Geometry: final body of the model. Coordinates: model frame, mm. Face numbers are marked on the shaded views. A direction names the side the tool comes from. Round coordinates to 2 decimals unless told otherwise and drop trailing zeros. Write each loop counter-clockwise with the first axis right and the second up, starting at its lowest first coordinate (ties: lowest second). Pieces come first, ordered by that corner, then holes. Notation, with made-up numbers: (76.25, 75) - (82.25, 75) arc R30 cw to (82.25, 112) - close; hole circle Ø7 at (33, 25.25). An arc over 180 degrees is marked (long way). Write each question's results on one line, items separated by ' | '.
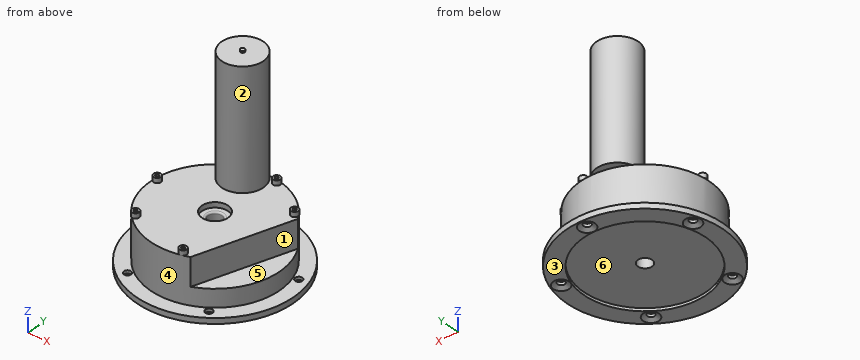
from build123d import *

# Parameters (mm, degrees)
FILLET1_R          = 1.524
SKETCH3_R          = 56.007
EXTRUDE1_DEPTH     = 2.6416
EXTRUDE3_REACH     = 7.08
SKETCH5_R          = 3.2639
CHAMFER1_SIZE      = 3.9878
CHAMFER1_SIZE2     = 2.302357403
EXTRUDE4_DEPTH     = 25.4
SKETCH7_R          = 19.05
EXTRUDE5_DEPTH     = 107.95
SKETCH9_R          = 3.3655
EXTRUDE6_DEPTH     = 4.445
SKETCH10_R         = 1.9685
EXTRUDE7_DEPTH     = 24.765
CUT_EXTRUDE1_START = 1.5875
SKETCH15_R         = 1.9685
CUT_EXTRUDE1_DEPTH = 24.1775


with BuildPart() as part:
    # Sketch2 → Revolve1 (revolve)
    with BuildSketch(Plane(origin=(0, 0, 0), x_dir=(0, 0, -1), z_dir=(1, 0, 0))):
        Polygon((0, 6.477), (0, 71.8185), (-5.08, 71.8185), (-5.08, 58.9915), (-46.609, 58.9915), (-46.609, 11.938), (-41.8465, 11.938), (-41.8465, 6.477), align=None)
    revolve(axis=Axis((0, 0, 46.609), (0, 0, -1)))

    # Fillet1
    fillet1_edges = [part.edges().sort_by_distance(p)[0] for p in [
        (0, -6.477, 41.8465),
    ]]
    fillet(fillet1_edges, radius=FILLET1_R)

    # Sketch3 → Extrude1 (cut)
    with BuildSketch(Plane(origin=(0, 0, 0), x_dir=(-1, 0, 0), z_dir=(0, 0, -1))):
        Circle(SKETCH3_R)
    extrude(amount=-EXTRUDE1_DEPTH, mode=Mode.SUBTRACT)

    # Sketch5 → Extrude3 (cut, up to next)
    with BuildSketch(Plane.XY.offset(5.08), mode=Mode.PRIVATE) as extrude3_sk1:
        with Locations((0, 63.5)):
            Circle(SKETCH5_R)
    extrude3_tool1 = extrude(extrude3_sk1.sketch, amount=-EXTRUDE3_REACH, mode=Mode.PRIVATE) & part.part
    add(extrude3_tool1.solids().sort_by_distance((0, 63.5, 5.08))[0], mode=Mode.SUBTRACT)
    # Sketch5 → Extrude3 (cut, up to next)
    with BuildSketch(Plane.XY.offset(5.08), mode=Mode.PRIVATE) as extrude3_sk2:
        with Locations((60.392088785, 19.622579143)):
            Circle(SKETCH5_R)
    extrude3_tool2 = extrude(extrude3_sk2.sketch, amount=-EXTRUDE3_REACH, mode=Mode.PRIVATE) & part.part
    add(extrude3_tool2.solids().sort_by_distance((60.392089, 19.622579, 5.08))[0], mode=Mode.SUBTRACT)
    # Sketch5 → Extrude3 (cut, up to next)
    with BuildSketch(Plane.XY.offset(5.08), mode=Mode.PRIVATE) as extrude3_sk3:
        with Locations((37.324363521, -51.372579143)):
            Circle(SKETCH5_R)
    extrude3_tool3 = extrude(extrude3_sk3.sketch, amount=-EXTRUDE3_REACH, mode=Mode.PRIVATE) & part.part
    add(extrude3_tool3.solids().sort_by_distance((37.324364, -51.372579, 5.08))[0], mode=Mode.SUBTRACT)
    # Sketch5 → Extrude3 (cut, up to next)
    with BuildSketch(Plane.XY.offset(5.08), mode=Mode.PRIVATE) as extrude3_sk4:
        with Locations((-37.324363521, -51.372579143)):
            Circle(SKETCH5_R)
    extrude3_tool4 = extrude(extrude3_sk4.sketch, amount=-EXTRUDE3_REACH, mode=Mode.PRIVATE) & part.part
    add(extrude3_tool4.solids().sort_by_distance((-37.324364, -51.372579, 5.08))[0], mode=Mode.SUBTRACT)
    # Sketch5 → Extrude3 (cut, up to next)
    with BuildSketch(Plane.XY.offset(5.08), mode=Mode.PRIVATE) as extrude3_sk5:
        with Locations((-60.392088785, 19.622579143)):
            Circle(SKETCH5_R)
    extrude3_tool5 = extrude(extrude3_sk5.sketch, amount=-EXTRUDE3_REACH, mode=Mode.PRIVATE) & part.part
    add(extrude3_tool5.solids().sort_by_distance((-60.392089, 19.622579, 5.08))[0], mode=Mode.SUBTRACT)

    # Chamfer1
    chamfer1_edges = [part.edges().sort_by_distance(p)[0] for p in [
        (-3.2639, 63.5, 0),
        (57.128188785, 19.622579143, 0),
        (34.060463521, -51.372579143, 0),
        (-40.588263521, -51.372579143, 0),
        (-63.655988785, 19.622579143, 0),
    ]]
    chamfer1_side = [part.faces().sort_by_distance(p)[0] for p in [
        (0, -69.787166065, 0),
    ]]
    chamfer(chamfer1_edges, length=CHAMFER1_SIZE, length2=CHAMFER1_SIZE2, reference=chamfer1_side[0])

    # Sketch6 → Extrude4 (cut)
    with BuildSketch(Plane.XY.offset(46.609)):
        Polygon((50.54556585, 30.416160921), (23.014050942, -54.317129264), (47.170886456, -62.166160921), (74.702401364, 22.567129264), align=None)
    extrude(amount=-EXTRUDE4_DEPTH, mode=Mode.SUBTRACT)

    # Sketch7 → Extrude5 (add)
    with BuildSketch(Plane.XY.offset(46.609)):
        with Locations((-12.023794238, 44.70269952)):
            Circle(SKETCH7_R)
    extrude(amount=EXTRUDE5_DEPTH)

    # Sketch9 → Extrude6 (add)
    with BuildSketch(Plane.XY.offset(46.609)):
        with Locations((45.289737364, 33.164222372)):
            Circle(SKETCH9_R)
        Polygon((46.260636305, 31.696529201), (47.046246406, 33.271198934), (46.075347464, 34.738892106), (44.318838422, 34.631915543), (43.533228322, 33.057245809), (44.504127263, 31.589552638), align=None, mode=Mode.SUBTRACT)
        with Locations((10.504871796, 55.142303403)):
            Circle(SKETCH9_R)
        Polygon((12.215906667, 54.731052055), (11.716543346, 56.418477394), (10.005508475, 56.829728741), (8.793836925, 55.55355475), (9.293200246, 53.866129412), (11.004235117, 53.454878064), align=None, mode=Mode.SUBTRACT)
        with Locations((15.674172573, -53.901264087)):
            Circle(SKETCH9_R)
        Polygon((13.962925135, -54.311630029), (15.173936185, -55.588430811), (16.885183622, -55.178064869), (17.38542001, -53.490898144), (16.174408961, -52.214097362), (14.463161523, -52.624463305), align=None, mode=Mode.SUBTRACT)
        with Locations((-56.011502863, 3.706413765)):
            Circle(SKETCH9_R)
        Polygon((-55.811839617, 5.454813773), (-57.425830063, 4.753527212), (-57.625493309, 3.005127204), (-56.211166109, 1.958013757), (-54.597175663, 2.659300318), (-54.397512417, 4.407700326), align=None, mode=Mode.SUBTRACT)
        with Locations((-39.544118158, -39.840791598)):
            Circle(SKETCH9_R)
        Polygon((-40.732661518, -38.543050222), (-41.262266837, -40.221229654), (-40.073723476, -41.51897103), (-38.355574797, -41.138532974), (-37.825969478, -39.460353542), (-39.014512839, -38.162612166), align=None, mode=Mode.SUBTRACT)
    extrude(amount=EXTRUDE6_DEPTH)

    # Sketch10 → Extrude7 (add)
    with BuildSketch(Plane.XY.offset(154.559)):
        with Locations((-12.023794238, 44.70269952)):
            Circle(SKETCH10_R)
    extrude(amount=EXTRUDE7_DEPTH)

    # Sketch15 → Cut-Extrude1 (cut, through all)
    with BuildSketch(Plane.XY.offset(154.559).offset(CUT_EXTRUDE1_START)):
        with Locations((-12.023794238, 44.70269952)):
            Circle(SKETCH15_R)
    extrude(amount=CUT_EXTRUDE1_DEPTH, mode=Mode.SUBTRACT)


solid = part.part
Q1. Mould query, pull axis X, two halves, no side actions, for the marked faces 4, 5 and 6. Classes: pulls with the +X half, pulls with the -X half, needs draft (parallel to the pull), parting line crosses it, or undercut.
Answer block:
face 4: parting line crosses it | face 5: needs draft | face 6: undercut
Q2. Section query C-C, the plane z = 88.5. Return loops of the section in (x, y).
Answer block:
outline: circle Ø38.1 at (-12.02, 44.7)
Q3. Access query for the marked faces 1, 2 and 3. Directions: +Z, -Z, +X, -X, +Y, -Y. A direction counts if a zero-diameter tool reaches every point of the face in a straight line with its end or side. Return the directions, or none.
Answer block:
face 1: +Z, +X, -Y | face 2: +Z | face 3: -Z, +X, -X, +Y, -Y
Q4. Section query B-B, the plane x = -49.5. Return loops of the section in (y, z), plus the area to 3 significant figures.
Answer block:
outline: (-52.04, 0) - (-26.2, 0) - (-26.2, 2.64) - (26.2, 2.64) - (26.2, 0) - (52.04, 0) - (52.04, 5.08) - (32.09, 5.08) - (32.09, 46.61) - (-32.09, 46.61) - (-32.09, 5.08) - (-52.04, 5.08) - close | area: 3,060 mm2
Q5. Section query A-A, the plane z = 30.5. Return loops of the section in (x, y), plus the area to 3 significant figures.
Answer block:
outline: (23.01, -54.32) - (50.55, 30.42) arc R58.99 ccw (long way) to start; hole circle Ø12.95 at (0, 0) | area: 9,550 mm2
Q6. Ray query, line 1 along Z through (x, y) = (-25, -19.5); line 2 along Z through (x, y) = (-64, -22); line 3 along X through (y, z) = (0, 45.2). Return the intervals inside material, ascending.
Answer block:
line 1: 2.64 to 46.61 | line 2: 0 to 5.08 | line 3: -58.99 to -11.94, 11.94 to 40.66
Q7. Pin query (flat end, axial travel): pin 1 (6 mm diameter, centred on x = -26.5, z = 73, fed in from +Y); pin 2 (0.5 mm diameter, centred on x = -59, y = 3.5, fed in from -Z); pin 3 (10.5 mm diameter, centred on x = 60.39, y = 19.62, fed in from -Z); pin 4 (5.5 mm diameter, centred on x = -40, y = -38.5, fed in from +Z). Return the tip coordinate at first contact, or that it passes through.
Answer block:
pin 1: y = 59.91 | pin 2: z = 0 | pin 3: z = 1.15 | pin 4: z = 51.05
